Model file for the job. Use its own axes, mm. A direction names the side the tool comes from. Coordinates: 2 decimals unless noted, no trailing zeros. Loops run counter-clockwise (first coordinate to the right, second up) from the corner with the lowest first, then second, coordinate; pieces in that order, holes last. Notation, with made-up numbers: (21.25, 51) -> (76.25, 51) arc R34 cw to (76.25, 90) -> close; hole circle Ø5 at (27, 83.5). An arc over 180 degrees is marked (long way). Use one line per item in the form item = value.
```python
from build123d import *

# Parameters (mm, degrees)
F1_DEPTH = 6.35
F3_DEPTH = 1.27
F4_R     = 3.3782
F5_DEPTH = 6.351
F6_R     = 3.175


with BuildPart() as f1:
    # F0 (on Top) → F1 (new body)
    with BuildSketch(Plane.XY):
        with BuildLine():
            Line((19.05, 25.4), (0, 25.4))
            Line((0, 25.4), (0, -25.4))
            Line((0, -25.4), (19.05, -25.4))
            Line((19.05, -25.4), (25.565484, -43.301144))
            Line((25.565484, -43.301144), (42.757881, -35.096026))
            ThreePointArc((42.757881, -35.096026), (34.812296, 0), (42.757881, 35.096026))
            Line((42.757881, 35.096026), (25.565484, 43.301144))
            Line((25.565484, 43.301144), (19.05, 25.4))
        make_face()
    extrude(amount=F1_DEPTH)

    # F2 (on face) → F3 (cut)
    with BuildSketch(Plane(origin=(0, 0, 0), x_dir=(1, 0, 0), z_dir=(0, 0, -1))):
        with BuildLine():
            Line((36.051805, 38.296519), (32.272126, 40.100381))
            ThreePointArc((32.272126, 40.100381), (21.04302, 0), (32.272126, -40.100381))
            Line((32.272126, -40.100381), (36.051805, -38.296519))
            ThreePointArc((36.051805, -38.296519), (25.20862, 0), (36.051805, 38.296519))
        make_face()
    extrude(amount=-F3_DEPTH, mode=Mode.SUBTRACT)

    # F4 (on face) → F5 (cut, through all)
    with BuildSketch(Plane.XY.offset(6.35)):
        with Locations((6.985, 15.875)):
            Circle(F4_R)
        with Locations((6.985, -15.875)):
            Circle(F4_R)
    extrude(amount=-F5_DEPTH, mode=Mode.SUBTRACT)

    # F6
    f6_edges = [f1.edges().sort_by_distance(p)[0] for p in [
        (0, -25.4, 3.175),
        (19.05, -25.4, 3.175),
        (25.565484, -43.301144, 3.175),
        (42.757881, -35.096026, 3.175),
        (0, 25.4, 3.175),
        (42.757881, 35.096026, 3.175),
        (25.565484, 43.301144, 3.175),
        (19.05, 25.4, 3.175),
    ]]
    fillet(f6_edges, radius=F6_R)


solid = f1.part
```
Q1. Band-saw the part on A-A, the plane x = 4.5. Write the cut outline in (y, z).
Result:
outline = (-25.4, 0) -> (-18.16, 0) -> (-18.16, 6.35) -> (-25.4, 6.35) -> close; (-13.59, 0) -> (13.59, 0) -> (13.59, 6.35) -> (-13.59, 6.35) -> close; (18.16, 0) -> (25.4, 0) -> (25.4, 6.35) -> (18.16, 6.35) -> close
Q2. Band-saw the part on B-B, the plane y = -29.5. Write the cut outline in (x, z).
Result:
outline = (20.54, 0) -> (26.9, 0) -> (26.9, 1.27) -> (31.43, 1.27) -> (31.43, 0) -> (40.34, 0) -> (40.34, 6.35) -> (20.54, 6.35) -> close
Q3. Which spindle directions (+Z, -Z, +X, -X, +Y, -Y) get a long thin tool onto all of the face, cutting with end or side? Do faces 1 (the face through (10, 25.4, 3)), 2 (the face through (12, 1, 0)), 3 (the face through (25, -3, 1.27)). Say none if no direction does.
Result:
face_1 = +Z, -Z, -X, +Y
face_2 = -Z, +X, -X, +Y, -Y
face_3 = -Z
Q4. Wall check: line 1 along X through (y, z) = (-16.5, 5.5); line 2 along Z through (x, y) = (23.5, 10); line 3 along X through (y, z) = (-17, 3.25). Give the ranges that are in metal, low to high.
Result:
line_1 = 0 to 3.67, 10.3 to 36.5
line_2 = 1.27 to 6.35
line_3 = 0 to 3.8, 10.17 to 36.61
Q5. Band-saw the part on D-D, the plane x = 26. Write the cut outline in (y, z).
Result:
outline = (-41.8, 0) -> (-27.22, 0) -> (-27.22, 1.27) -> (-10.72, 1.27) -> (-10.72, 0) -> (10.72, 0) -> (10.72, 1.27) -> (27.22, 1.27) -> (27.22, 0) -> (41.8, 0) -> (41.8, 6.35) -> (-41.8, 6.35) -> close
Q6. Mould opens along Y. For faces 4 (the face through (25.21, 0.56, 0.63)), 5 (the face through (0, 0, 3)), 6 (the face through (21.045, -0.59, 0.626)), 7 (the face through (22.12, 33.84, 3.13)) say: released by +Y, released by -Y, zero draft, split by the parting line, or undercut.
Result:
face_4 = undercut
face_5 = zero draft
face_6 = undercut
face_7 = released by +Y
Q7. Pin check, flat tips, straight feed: pin 1 Ø1 at (x, z) = (15, 5) entering from +Y; pin 2 Ø3 at (x, z) = (9, 2.5) entering from -Y; pin 3 Ø3 at (x, y) = (31, -32.5) entering from -Z. Stop position of each tip, or through.
Result:
pin_1 = 25.4
pin_2 = -25.4
pin_3 = 1.27
Q8. Band-saw the part on C-C, the plane z = 2.75. State how many separate pieces and enclosed holes the cut face has, and give its area (3 significant figures).
Result:
separate_pieces = 1
enclosed_holes = 2
area = 2,300 mm2
